```python
from build123d import *

# Parameters (mm, degrees)
SKETCH_1_R          = 2.4
EXTRUDE_1_DEPTH     = 5
SKETCH_2_R          = 13.5
EXTRUDE_2_DEPTH     = 5
SKETCH_3_R          = 13.5
SKETCH_3_R_2        = 12
EXTRUDE_3_DEPTH     = 2
SKETCH_4_R          = 5
SKETCH_4_R_2        = 4
EXTRUDE_4_DEPTH     = 6
SKETCH_5_R          = 6
CUT_EXTRUDE_1_DEPTH = 7
SKETCH_6_R          = 4
CUT_EXTRUDE_2_DEPTH = 13
SKETCH_7_R          = 10.5
SKETCH_7_R_2        = 9.5
EXTRUDE_5_DEPTH     = 1
SKETCH_8_R          = 2
CUT_EXTRUDE_3_DEPTH = 3


with BuildPart() as part:
    # 草图1 → 凸台-拉伸1 (new body)
    with BuildSketch(Plane.XY):
        with BuildLine():
            Line((-23.650515621, 4.155817481), (-14.755275826, 6.353883931))
            ThreePointArc((-14.755275826, 6.353883931), (-12.096586798, 7.435137426), (-9.854528975, 9.227039541))
            ThreePointArc((-9.854528975, 9.227039541), (0.022244584, 13.499981673), (9.884883075, 9.19451394))
            ThreePointArc((9.884883075, 9.19451394), (12.1232727, 7.393904675), (14.781202624, 6.30395497))
            Line((14.781202624, 6.30395497), (23.663193746, 4.083009896))
            ThreePointArc((23.663193746, 4.083009896), (24.012837039, -0.036951588), (23.650515621, -4.155817481))
            Line((23.650515621, -4.155817481), (14.755275826, -6.353883931))
            ThreePointArc((14.755275826, -6.353883931), (12.096586798, -7.435137426), (9.854528975, -9.227039541))
            ThreePointArc((9.854528975, -9.227039541), (-0.168191571, -13.498952241), (-10.081364571, -8.978646244))
            ThreePointArc((-10.081364571, -8.978646244), (-12.295346053, -7.120754011), (-14.948193848, -5.973637572))
            Line((-14.948193848, -5.973637572), (-23.740665236, -3.605346339))
            ThreePointArc((-23.740665236, -3.605346339), (-24.011245735, 0.278902058), (-23.650515621, 4.155817481))
        make_face()
        with Locations((18.5, 0)):
            Circle(SKETCH_1_R, mode=Mode.SUBTRACT)
        with Locations((-18.5, 0)):
            Circle(SKETCH_1_R, mode=Mode.SUBTRACT)
    extrude(amount=EXTRUDE_1_DEPTH)

    # 草图2 → 凸台-拉伸2 (add)
    with BuildSketch(Plane.XY.offset(5)):
        Circle(SKETCH_2_R)
    extrude(amount=EXTRUDE_2_DEPTH)

    # 草图3 → 凸台-拉伸3 (add)
    with BuildSketch(Plane.XY.offset(10)):
        Circle(SKETCH_3_R)
        Circle(SKETCH_3_R_2, mode=Mode.SUBTRACT)
    extrude(amount=EXTRUDE_3_DEPTH)

    # 草图4 → 凸台-拉伸4 (add)
    with BuildSketch(Plane.XY.offset(10)):
        Circle(SKETCH_4_R)
        Circle(SKETCH_4_R_2, mode=Mode.SUBTRACT)
    extrude(amount=EXTRUDE_4_DEPTH)

    # 草图5 → 切除-拉伸1 (cut)
    with BuildSketch(Plane.XY.offset(5)):
        with Locations((-18.5, 0)):
            Circle(SKETCH_5_R)
        with Locations((18.5, 0)):
            Circle(SKETCH_5_R)
    extrude(amount=CUT_EXTRUDE_1_DEPTH, mode=Mode.SUBTRACT)

    # 草图6 → 切除-拉伸2 (cut)
    with BuildSketch(Plane.XY.offset(10)):
        Circle(SKETCH_6_R)
    extrude(amount=-CUT_EXTRUDE_2_DEPTH, mode=Mode.SUBTRACT)

    # 草图7 → 凸台-拉伸5 (add)
    with BuildSketch(Plane.XY.offset(10)):
        Circle(SKETCH_7_R)
        Circle(SKETCH_7_R_2, mode=Mode.SUBTRACT)
    extrude(amount=EXTRUDE_5_DEPTH)

    # 草图8 → 切除-拉伸3 (cut)
    with BuildSketch(Plane.ZY.offset(5)):
        with Locations((13, 0)):
            Circle(SKETCH_8_R)
    extrude(amount=-CUT_EXTRUDE_3_DEPTH, mode=Mode.SUBTRACT)


solid = part.part
```
Source: CAD feature listing. Evaluate the final solid. Frame: model axes, mm. A direction names the side the tool comes from. Give positions to 0.01 mm unless a question says otherwise; leave off trailing zeros. Loops run counter-clockwise (first coordinate to the right, second up) from the corner with the lowest first, then second, coordinate; pieces in that order, holes last. Notation, with made-up numbers: (49.25, -15.5) -> (87.25, -15.5) arc R16 ccw to (87.25, -2.5) -> close; hole circle Ø10 at (-21, 24.5). An arc over 180 degrees is marked (long way). Put each result on its own line as item: value. Start each with the question number.
1) Contact query for flat-ended pins moving along their axis: P1, Ø7.5, axis at x = 18.5, y = 0, coming from the -Z side; P2, Ø7, axis at x = -14, y = 4.5, coming from the +Z side; P3, Ø4, axis at y = -0.5, z = 11, coming from the +X side; P4, Ø2, axis at y = 2.5, z = 13.5, coming from the -X side. Output: stop coordinate, or through.
2) Material intervals for probe 1 along Y at (x, z) = (0, 11.4); probe 2 along Y at (x, z) = (0, 12.5); probe 3 along X at (y, z) = (0, 5.25), sorted ascending.
3) Reachability of faces 4 (the face through (12.131, -7.415, 2.465)), 5 (the face through (12.5, 0, 8.5)), 6 (the face through (4.38, -8.43, 10.49)), 7 (the face through (0.257, 13.498, 7.249)) from +Z, -Z, +X, -X, +Y, -Y: full face, straight path, thin tool, end or side. Return the list, or none.
4) Cut plane D-D (y = 8). Return loops of the section in (x, z), then the cut area to 3 significant figures.
5) Draft query along Z for faces 1 (the face through (0, -11, 10)), 2 (the face through (-4.243, 0.088, 11.002)), 3 (the face through (-5, 0, 0)). Return one class per face: released by +Z, released by -Z, zero draft, split by the parting line, or undercut.
6) Cut plane B-B (x = -18.5). Return loops of the section in (y, z), then the cut area to 3 significant figures.
7) Cut plane C-C (z = 8.75). Return loops of the section in (x, y), then the cut area to 3 significant figures.
8) Cut plane A-A (z = 4). Return loops of the section in (x, y), then the cut area to 3 significant figures.
Results are:
1. P1: stops at z = 0
1. P2: stops at z = 12
1. P3: stops at x = 13.05
1. P4: stops at x = -4.71
2. probe 1: y = -13.5 to -12, -5 to -4, 4 to 5, 12 to 13.5
2. probe 2: y = -5 to -4, 4 to 5
2. probe 3: x = -12.5 to -4, 4 to 12.5
3. face 4: +Z, -Z, +X, -Y
3. face 5: +Z, +X
3. face 6: +Z
3. face 7: +Z, +Y
4. outline: (-11.24, 0) -> (11.21, 0) -> (11.21, 5) -> (10.87, 5) -> (10.87, 12) -> (8.94, 12) -> (8.94, 10) -> (6.8, 10) -> (6.8, 11) -> (5.12, 11) -> (5.12, 10) -> (-5.12, 10) -> (-5.12, 11) -> (-6.8, 11) -> (-6.8, 10) -> (-8.94, 10) -> (-8.94, 12) -> (-10.87, 12) -> (-10.87, 5) -> (-11.24, 5) -> close
4. area: 232 mm2
5. face 1: released by +Z
5. face 2: undercut
5. face 3: released by -Z
6. outline: (-5.02, 0) -> (-2.4, 0) -> (-2.4, 5) -> (-5.02, 5) -> close; (2.4, 0) -> (5.43, 0) -> (5.43, 5) -> (2.4, 5) -> close
6. area: 28.2 mm2
7. outline: (-13.2, -2.82) arc R13.5 ccw to (13.2, -2.82) arc R6 cw to (13.2, 2.82) arc R13.5 ccw to (-13.2, 2.82) arc R6 cw to start; hole circle Ø8 at (0, 0)
7. area: 515 mm2
8. outline: (-23.74, -3.61) -> (-14.95, -5.97) arc R10 cw to (-10.08, -8.98) arc R13.5 ccw to (9.85, -9.23) arc R10 cw to (14.76, -6.35) -> (23.65, -4.16) arc R24.01 ccw to (23.66, 4.08) -> (14.78, 6.3) arc R10 cw to (9.88, 9.19) arc R13.5 ccw to (-9.85, 9.23) arc R10 cw to (-14.76, 6.35) -> (-23.65, 4.16) arc R24.01 ccw to start; hole circle Ø4.8 at (-18.5, 0); hole circle Ø8 at (0, 0); hole circle Ø4.8 at (18.5, 0)
8. area: 726 mm2
